```python
from build123d import *

# Parameters (mm, degrees)
BOSS_EXTRUDE1_DEPTH = 10
DRAFT1_ANGLE        = 15


with BuildPart() as part:
    # Sketch1 → Boss-Extrude1 (new body)
    with BuildSketch(Plane(origin=(0, 0, 0), x_dir=(1, 0, 0), z_dir=(0, 1, 0))):
        Polygon((-75, 30), (75, 30), (75, 10), (65, 10), (65, -10), (75, -10), (75, -30), (-75, -30), (-75, -10), (-65, -10), (-65, 10), (-75, 10), align=None)
    extrude(amount=BOSS_EXTRUDE1_DEPTH)

    # Draft1
    draft1_faces = [part.faces().sort_by_distance(p)[0] for p in [
        (0, 5, 30),
        (0, 5, -30),
    ]]
    draft(draft1_faces, Plane.ZX.offset(10), DRAFT1_ANGLE)


solid = part.part
```
Geometry: final body of the model. Coordinates: model frame, mm. A direction names the side the tool comes from. Round coordinates to 2 decimals unless told otherwise and drop trailing zeros. Order: outer loops, then holes, each group sorted by start corner. A loop starts at its lowest first (then second) coordinate and runs counter-clockwise, first axis right, second up. Notation, with made-up numbers: M 54,71 L 80,71 A21 cw 80,96 Z; hole C 74,8 d5. An arc over 180 degrees is marked long. One line per item, written item: value.
(1) Cut plane C-C (z = 2.5). Return the cut outline in (x, y).
Result sheet:
outline: M -65,0 L 65,0 L 65,10 L -65,10 Z
(2) Pull-direction query (Z, two-part tool) for faces 1 (the flat face through (-70, 5, -10)), 2 (the flat face through (1.05, 4.93, 31.36)), 3 (the flat face through (1, 10, 0)), 4 (the flat face through (-70, 5, 10)); classes: pulls with the +Z half, pulls with the -Z half, needs draft (parallel to the pull), parting line crosses it, or undercut.
Result sheet:
face 1: undercut
face 2: pulls with the +Z half
face 3: needs draft
face 4: undercut
(3) Cut plane B-B (x = 29). Return the cut outline in (y, z), and give its area (3 significant figures).
Result sheet:
outline: M 0,-32.68 L 10,-30 L 10,30 L 0,32.68 Z
area: 627 mm2
(4) Pin query (flat end, axial travel): P1, Ø5, axis at x = -56, y = 4.5, coming from the +Z side; P2, Ø4, axis at y = 5, z = -3.5, coming from the -X side; P3, Ø5, axis at y = 4.5, z = 0.5, coming from the +X side. Return the tip coordinate at first contact, or that it passes through.
Result sheet:
P1: z = 32.14
P2: x = -65
P3: x = 65
(5) Reachability of faces 5 (the flat face through (-65, 5, 0)), 6 (the flat face through (70, 5, -10)), 7 (the flat face through (1, 0, 0)) from +Z, -Z, +X, -X, +Y, -Y: full face, straight path, thin tool, end or side. Return the list, or none.
Result sheet:
face 5: -X, +Y, -Y
face 6: +X, +Y, -Y
face 7: +Z, -Z, +X, -X, -Y
(6) Line query: probe 1 along X at (y, z) = (2.25, 1); probe 2 along Z at (x, y) = (-42, 3.5); probe 3 along Z at (x, y) = (-30, 5.5). Output: solid intervals per line, ascending. Write a range as [from, to].
Result sheet:
probe 1: [-65, 65]
probe 2: [-31.74, 31.74]
probe 3: [-31.21, 31.21]
(7) Cut plane A-A (y = 5.25). Return the cut outline in (x, z).
Result sheet:
outline: M -75,-31.27 L 75,-31.27 L 75,-10 L 65,-10 L 65,10 L 75,10 L 75,31.27 L -75,31.27 L -75,10 L -65,10 L -65,-10 L -75,-10 Z
